Geometry check sheet. Reference: the model listing, model coordinates, mm. Face numbers are marked on the shaded views. A direction names the side the tool comes from. Give positions to 0.01 mm unless a question says otherwise; leave off trailing zeros. Loops run counter-clockwise (first coordinate to the right, second up) from the corner with the lowest first, then second, coordinate; pieces in that order, holes last. Notation, with made-up numbers: (16.5, 54) -> (66.5, 54) arc R7 cw to (66.5, 61) -> close; hole circle Ø1 at (-19.5, 29.5). An arc over 180 degrees is marked (long way). One line per question, with ' | ' between items.
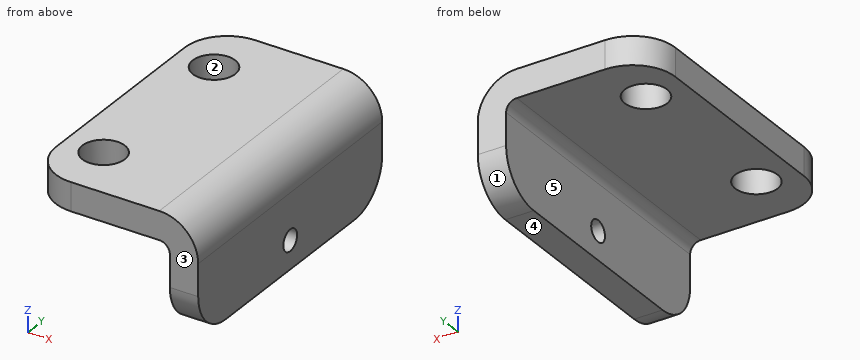
from build123d import *

# Parameters (mm, degrees)
BOSS_EXTRUDE1_DEPTH = 20
FILLET1_R           = 3
SKETCH3_R           = 1.5
CUT_EXTRUDE1_DEPTH  = 24.600847442
SKETCH4_R           = 0.75
CUT_EXTRUDE2_DEPTH  = 24.430749028
SCALE1_SCALE        = 1.9


with BuildPart() as part:
    # Sketch2 → Boss-Extrude1 (new body)
    with BuildSketch(Plane(origin=(0, 0, 0), x_dir=(1, 0, 0), z_dir=(0, 1, 0))):
        with BuildLine():
            Line((-1, 7), (1, 7))
            Line((1, 7), (1, 1.75))
            ThreePointArc((1, 1.75), (0.194543648, -0.194543648), (-1.75, -1))
            Line((-1.75, -1), (-11, -1))
            Line((-11, -1), (-11, 1))
            Line((-11, 1), (-1.75, 1))
            ThreePointArc((-1.75, 1), (-1.219669914, 1.219669914), (-1, 1.75))
            Line((-1, 1.75), (-1, 7))
        make_face()
    extrude(amount=BOSS_EXTRUDE1_DEPTH)

    # Fillet1
    fillet1_edges = [part.edges().sort_by_distance(p)[0] for p in [
        (-11, 0, 0),
        (-11, 20, 0),
        (0, 20, -7),
        (0, 0, -7),
    ]]
    fillet(fillet1_edges, radius=FILLET1_R)

    # Sketch3 → Cut-Extrude1 (cut, through all)
    with BuildSketch(Plane(origin=(0, 0, -1), x_dir=(-1, 0, 0), z_dir=(0, 0, -1))):
        with Locations((8.28, 16)):
            Circle(SKETCH3_R)
        with Locations((8.28, 4)):
            Circle(SKETCH3_R)
    extrude(amount=-CUT_EXTRUDE1_DEPTH, mode=Mode.SUBTRACT)

    # Sketch4 → Cut-Extrude2 (cut, through all)
    with BuildSketch(Plane.ZY.offset(1)):
        with Locations((-5, 10)):
            Circle(SKETCH4_R)
    extrude(amount=-CUT_EXTRUDE2_DEPTH, mode=Mode.SUBTRACT)


with BuildPart() as part_1:
    # Scale1: scaled about (-3.269699992, 10, -1.413989503)
    add(part.part.scale(SCALE1_SCALE).moved(Location((2.942729993, -9, 1.272590553))))


solid = part_1.part
Item 1: Depth check by flat-ended pin: pin 1 Ø6.5 at (x, y) = (-12.79, -1.4) entering from -Z; pin 2 Ø4 at (x, y) = (0, 5) entering from +Z; pin 3 Ø6 at (y, z) = (-5, -3.5) entering from -X. Enter the tip coordinate at first touch or a pass-through.
Result:
pin 1: z = -0.63 | pin 2: z = 3.17 | pin 3: x = -17.9
Item 2: Sectioned sample at A-A (y = -1.4). Record the cut outline in (x, z) (3 decimals), plus the area to 3 significant figures.
Result:
outline: (-17.957, -0.627) -> (-15.639, -0.627) -> (-15.639, 3.173) -> (-17.957, 3.173) -> close; (-9.939, -0.627) -> (-0.382, -0.627) arc R1.425 cw to (1.043, -2.052) -> (1.043, -12.027) -> (4.843, -12.027) -> (4.843, -2.052) arc R5.225 ccw to (-0.382, 3.173) -> (-9.939, 3.173) -> close | area: 103 mm2
Item 3: Sectioned sample at B-B (x = -15). Record the cut outline in (y, z).
Result:
outline: (-8.3, -0.63) -> (-3.2, -0.63) -> (-3.2, 3.17) -> (-8.3, 3.17) -> close; (0.4, -0.63) -> (19.6, -0.63) -> (19.6, 3.17) -> (0.4, 3.17) -> close; (23.2, -0.63) -> (28.3, -0.63) -> (28.3, 3.17) -> (23.2, 3.17) -> close
Item 4: Release check for a two-part mould opening along Y. For the marked faces 1, 2 and 3 record: pulls with the +Y half, pulls with the -Y half, needs draft (parallel to the pull), parting line crosses it, or undercut.
Result:
face 1: pulls with the +Y half | face 2: undercut | face 3: pulls with the -Y half
Item 5: Scan lines: probe 1 along Z at (x, y) = (-3, 11.5); probe 2 along X at (y, z) = (6, -3.5); probe 3 along Y at (x, z) = (-14.5, 1.25). Record each from-to range of solid material in increasing order.
Result:
probe 1: -0.63 to 3.17 | probe 2: 1.04 to 4.84 | probe 3: -8.54 to -3.68, 0.88 to 19.12, 23.68 to 28.54
Item 6: Set-up check for the marked faces 4 and 5: record each of +Z, -Z, +X, -X, +Y, -Y from which the full face is reachable in a straight line by a thin tool's end or side.
Result:
face 4: -Z, +X, -X, +Y, -Y | face 5: -Z, -X, +Y, -Y
Item 7: Sectioned sample at D-D (y = 10). Record the cut outline in (x, z) (3 decimals), plus the area to 3 significant figures.
Result:
outline: (-17.957, -0.627) -> (-0.382, -0.627) arc R1.425 cw to (1.043, -2.052) -> (1.043, -6.802) -> (4.843, -6.802) -> (4.843, -2.052) arc R5.225 ccw to (-0.382, 3.173) -> (-17.957, 3.173) -> close; (1.043, -12.027) -> (4.843, -12.027) -> (4.843, -9.652) -> (1.043, -9.652) -> close | area: 114 mm2
Item 8: Sectioned sample at C-C (z = 0.5). Record the cut outline in (x, y), plus the area to 3 significant figures.
Result:
outline: (-17.96, -3.3) arc R5.7 ccw to (-12.26, -9) -> (4.18, -9) -> (4.18, 29) -> (-12.26, 29) arc R5.7 ccw to (-17.96, 23.3) -> close; hole circle Ø5.7 at (-12.79, -1.4); hole circle Ø5.7 at (-12.79, 21.4) | area: 776 mm2
